Here's the drawing with two shaded views (mm, measured from the low corner). I have some questions. A direction names the side the tool comes from. Give positions to 0.01 mm unless a question says otherwise; leave off trailing zeros. Loops run counter-clockwise (first coordinate to the right, second up) from the corner with the lowest first, then second, coordinate; pieces in that order, holes last. Notation, with made-up numbers: M 45.25,50.5 L 99.25,50.5 A12 cw 99.25,65.5 Z; hole C -28.75,5.5 d7. An arc over 180 degrees is marked long. Put each result on its own line as item: value. Start each with the question number.
1) Imagine slicing it at C-C (z = 21). Write out the boundary of the cut face in (x, y).
2) For P1, Ø1, axis at y = 39.5, z = 23.5, coming from the -X side; P2, Ø11.5, axis at y = 31.5, z = 16.5, coming from the +X side; P3, Ø1.8, axis at x = 35, y = 35, coming from the -Z side; P4, Ø5, axis at x = 32.5, z = 18, coming from the +Y side, each with a flat end and sliding along its axis, tell me the tip position at first contact or that it passes through.
3) For the marked faces 1 and 2, which set-ups out of +Z, -Z, +X, -X, +Y, -Y let a thin tool reach every point of the face, with its end or its side?
4) Imagine slicing it at A-A (y = 35). Write out the boundary of the cut face in (x, z), then the cut area to 3 significant figures.
5) Please list where these lines run through material, in increasing order: line 1 along Y through (x, z) = (26, 2.25); line 2 along Z through (x, y) = (36, 7); line 3 along Y through (x, z) = (35, 24.4). Write a range as from..to.
6) Imagine slicing it at D-D (y = 17). Write out the boundary of the cut face in (x, z).
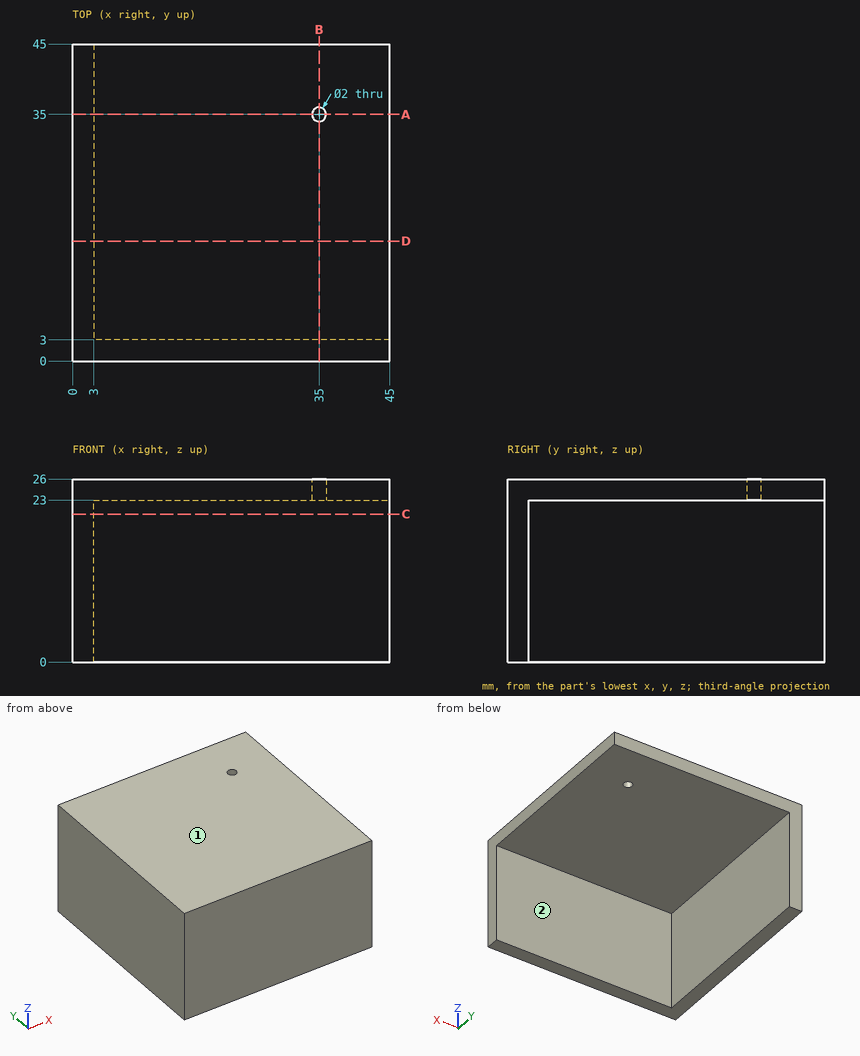
Recorded:
1. outline: M 0,0 L 45,0 L 45,3 L 3,3 L 3,45 L 0,45 Z
2. P1: x = 0
2. P2: x = 3
2. P3: through
2. P4: y = 3
3. face 1: +Z, +X, -X, +Y, -Y
3. face 2: -Z, +X, +Y
4. outline: M 0,0 L 3,0 L 3,23 L 34,23 L 34,26 L 0,26 Z; M 36,23 L 45,23 L 45,26 L 36,26 Z
4. area: 198 mm²
5. line 1: 0..3
5. line 2: 23..26
5. line 3: 0..34, 36..45
6. outline: M 0,0 L 3,0 L 3,23 L 45,23 L 45,26 L 0,26 Z
